Geometry check sheet. Reference: the model listing, model coordinates, mm. Face numbers are marked on the shaded views. A direction names the side the tool comes from. Give positions to 0.01 mm unless a question says otherwise; leave off trailing zeros. Write each loop counter-clockwise with the first axis right and the second up, starting at its lowest first coordinate (ties: lowest second). Pieces come first, ordered by that corner, then holes. Notation, with made-up numbers: (-28, 27.5) -> (11, 27.5) arc R7 cw to (11, 34.5) -> close; hole circle Ø1 at (40, 17). An arc over 180 degrees is marked (long way). Write item = value, one per line. Start each with the question number.
1. Thickness scan on line 1 along Y through (x, z) = (0, 0.5); line 2 along Z through (x, y) = (-21, -11.7); line 3 along X through (y, z) = (-10.25, 5). Record the ranges inside material, lowest first.
2. Cross-section at A-A, the plane z = 6. Record the cut outline in (x, y), plus the area to 3 significant figures.
3. Set-up check for the marked faces 1, 2, 3, 4 and 5: record each of +Z, -Z, +X, -X, +Y, -Y from which the full face is reachable in a straight line by a thin tool's end or side.
4. Depth check by flat-ended pin: P1, Ø5, axis at y = 3.5, z = 13, coming from the -X side; P2, Ø5, axis at x = 20, z = 5, coming from the +Y side; P3, Ø3, axis at x = 9, z = 5.5, coming from the +Y side; P4, Ø2.5, axis at x = -21, z = 6, coming from the +Y side. Enter the tip coordinate at first touch or a pass-through.
5. Cross-section at B-B, the plane x = 0. Record the cut outline in (y, z), plus the area to 3 significant figures.
6. Cross-section at D-D, the plane y = 3.25. Record the cut outline in (x, z).
7. Mould release check, pull along Z, two halves, no side actions. Record for the marked faces 6, 7, 8 and 9: pulls with the +Z half, pulls with the -Z half, needs draft (parallel to the pull), parting line crosses it, or undercut.
8. Cross-section at C-C, the plane z = 2.75. Record the cut outline in (x, y).
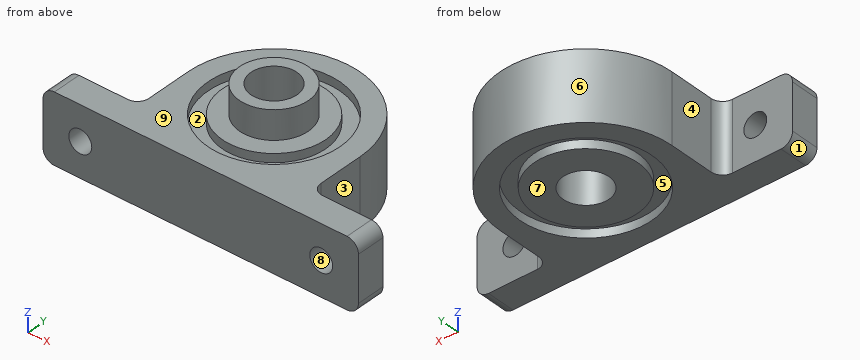
```python
from build123d import *

# Parameters (mm, degrees)
SKETCH_2_R          = 4
EXTRUDE_1_DEPTH     = 12
FILLET_1_R          = 2
SKETCH_3_R          = 2
CUT_EXTRUDE_1_DEPTH = 6
SKETCH_4_R          = 6
SKETCH_4_R_2        = 4
EXTRUDE_2_DEPTH     = 5
SKETCH_5_R          = 11.5
SKETCH_5_R_2        = 9
CUT_EXTRUDE_2_DEPTH = 1.5


with BuildPart() as part:
    # 草图2 → 凸台-拉伸1 (new body)
    with BuildSketch(Plane.XY):
        with BuildLine():
            Line((0, -15), (-27.5, -15))
            Line((-27.5, -15), (-27.5, -10))
            Line((-27.5, -10), (-17, -10))
            ThreePointArc((-17, -10), (-15.585786438, -9.414213562), (-15, -8))
            Line((-15, -8), (-15, 0))
            ThreePointArc((-15, 0), (0, 15), (15, 0))
            Line((15, 0), (15, -8))
            ThreePointArc((15, -8), (15.585786438, -9.414213562), (17, -10))
            Line((17, -10), (27.5, -10))
            Line((27.5, -10), (27.5, -15))
            Line((27.5, -15), (0, -15))
        make_face()
        Circle(SKETCH_2_R, mode=Mode.SUBTRACT)
    extrude(amount=EXTRUDE_1_DEPTH)

    # 圆角1
    fillet_1_edges = [part.edges().sort_by_distance(p)[0] for p in [
        (27.5, -12.5, 0),
        (-27.5, -12.5, 0),
        (-27.5, -12.5, 12),
        (27.5, -12.5, 12),
    ]]
    fillet(fillet_1_edges, radius=FILLET_1_R)

    # 草图3 → 切除-拉伸1 (cut, through all)
    with BuildSketch(Plane(origin=(0, -10, 0), x_dir=(1, 0, 0), z_dir=(0, 1, 0))):
        with Locations((-21, -6)):
            Circle(SKETCH_3_R)
        with Locations((21, -6)):
            Circle(SKETCH_3_R)
    extrude(amount=-CUT_EXTRUDE_1_DEPTH, mode=Mode.SUBTRACT)

    # 草图4 → 凸台-拉伸2 (add)
    with BuildSketch(Plane.XY.offset(12)):
        Circle(SKETCH_4_R)
        Circle(SKETCH_4_R_2, mode=Mode.SUBTRACT)
    extrude(amount=EXTRUDE_2_DEPTH)

    # 草图5 → 切除-拉伸2 (cut)
    with BuildSketch(Plane.XY.offset(12)):
        Circle(SKETCH_5_R)
        Circle(SKETCH_5_R_2, mode=Mode.SUBTRACT)
    cut_extrude_2 = extrude(amount=-CUT_EXTRUDE_2_DEPTH, mode=Mode.SUBTRACT)

    # 镜向1: 切除-拉伸2 across plane
    add(cut_extrude_2.mirror(Plane.XY.offset(6)), mode=Mode.SUBTRACT)


solid = part.part
```
Answers:
q1.line_1 = -15 to -11.5, -9 to -4, 4 to 9, 11.5 to 15
q1.line_2 = 0 to 4, 8 to 12
q1.line_3 = -27.5 to -22.73, -19.27 to 19.27, 22.73 to 27.5
q2.outline = (-27.5, -15) -> (-23, -15) -> (-23, -10) -> (-27.5, -10) -> close; (-19, -15) -> (19, -15) -> (19, -10) -> (17, -10) arc R2 cw to (15, -8) -> (15, 0) arc R15 ccw to (-15, 0) -> (-15, -8) arc R2 cw to (-17, -10) -> (-19, -10) -> close; (23, -15) -> (27.5, -15) -> (27.5, -10) -> (23, -10) -> close; hole circle Ø8 at (0, 0)
q2.area = 840 mm^2
q3.face_1 = -Z, -X, +Y, -Y
q3.face_2 = +Z
q3.face_3 = +Z, -Z, +X, +Y
q3.face_4 = +Z, -Z, -X, +Y
q3.face_5 = -Z
q4.P1 = -14.95
q4.P2 = -10
q4.P3 = 12.99
q4.P4 = through
q5.outline = (-15, 0) -> (-11.5, 0) -> (-11.5, 1.5) -> (-9, 1.5) -> (-9, 0) -> (-4, 0) -> (-4, 17) -> (-6, 17) -> (-6, 12) -> (-9, 12) -> (-9, 10.5) -> (-11.5, 10.5) -> (-11.5, 12) -> (-15, 12) -> close; (4, 0) -> (9, 0) -> (9, 1.5) -> (11.5, 1.5) -> (11.5, 0) -> (15, 0) -> (15, 12) -> (11.5, 12) -> (11.5, 10.5) -> (9, 10.5) -> (9, 12) -> (6, 12) -> (6, 17) -> (4, 17) -> close
q5.area = 269 mm^2
q6.outline = (-14.64, 0) -> (-11.03, 0) -> (-11.03, 1.5) -> (-8.39, 1.5) -> (-8.39, 0) -> (-2.33, 0) -> (-2.33, 17) -> (-5.04, 17) -> (-5.04, 12) -> (-8.39, 12) -> (-8.39, 10.5) -> (-11.03, 10.5) -> (-11.03, 12) -> (-14.64, 12) -> close; (2.33, 0) -> (8.39, 0) -> (8.39, 1.5) -> (11.03, 1.5) -> (11.03, 0) -> (14.64, 0) -> (14.64, 12) -> (11.03, 12) -> (11.03, 10.5) -> (8.39, 10.5) -> (8.39, 12) -> (5.04, 12) -> (5.04, 17) -> (2.33, 17) -> close
q7.face_6 = needs draft
q7.face_7 = pulls with the -Z half
q7.face_8 = undercut
q7.face_9 = pulls with the +Z half
q8.outline = (-27.5, -15) -> (27.5, -15) -> (27.5, -10) -> (17, -10) arc R2 cw to (15, -8) -> (15, 0) arc R15 ccw to (-15, 0) -> (-15, -8) arc R2 cw to (-17, -10) -> (-27.5, -10) -> close; hole circle Ø8 at (0, 0)
